from build123d import *

# Parameters (mm, degrees)
SKETCH2_R          = 6.858
EXTRUDE1_DEPTH     = 10.414
EXTRUDE1_DRAFT     = -1.5
CUT_EXTRUDE7_DEPTH = 5.5626


with BuildPart() as part:
    # Sketch2 → Extrude1 (with draft: the straight prism first)
    with BuildSketch(Plane(origin=(-5.207, 0, 0), x_dir=(0, 0, -1), z_dir=(1, 0, 0))):
        Circle(SKETCH2_R)
    extrude(amount=EXTRUDE1_DEPTH)
    # Extrude1: the draft: its side faces are tilted about the plane it starts from
    extrude1_sides = [part.faces().sort_by_distance(p)[0] for p in [
        (0, 0, 6.858),
    ]]
    draft(extrude1_sides, Plane(origin=(-5.207, 0, 0), x_dir=(0, 0, -1), z_dir=(1, 0, 0)), EXTRUDE1_DRAFT)

    # Sketch6 → Cut-Extrude7 (cut)
    with BuildSketch(Plane(origin=(5.207, 0, 0), x_dir=(0, 0, -1), z_dir=(1, 0, 0))):
        Polygon((0, 3.666174209), (-3.175, 1.833087105), (-3.175, -1.833087105), (0, -3.666174209), (3.175, -1.833087105), (3.175, 1.833087105), align=None)
    extrude(amount=-CUT_EXTRUDE7_DEPTH, mode=Mode.SUBTRACT)


solid = part.part
Can you work these out from the model? Positions are in its coordinate system, mm. A direction names the side the tool comes from. Give positions to 0.01 mm unless a question says otherwise; leave off trailing zeros. Order: outer loops, then holes, each group sorted by start corner. A loop starts at its lowest first (then second) coordinate and runs counter-clockwise, first axis right, second up. Notation, with made-up numbers: M 67,65.25 L 86,65.25 A16 ccw 86,92.25 Z; hole C 77.5,-7 d7. An arc over 180 degrees is marked long. Use a Markdown table: item, result. Add a question column.
Item 1: For faces 5 (the flat face through (2, 0, -3.175)), 6 (the flat face through (5.207, -3.1, -1.5)), which set-ups out of +Z, -Z, +X, -X, +Y, -Y let a thin tool reach every point of the face, with its end or its side?
Item 2: Suppose I cut it at D-D (x = -1.5). List the corners of the cut face in (y, z) for me, then the cut area to 3 significant figures.
Item 3: Suppose I cut it at C-C (x = -3). List the corners of the cut face in (y, z) for me.
Item 4: Suppose I cut it at B-B (x = 2). List the corners of the cut face in (y, z) for me (3 decimals).
Item 5: Suppose I cut it at A-A (y = 0). List the corners of the cut face in (x, z) for me (3 decimals), then the cut area to 3 significant figures.
Item 6: We'd pull the mould along Z, two halves only. Please class faces 1 (the flat face through (-5.207, 0, 0)), 2 (the flat face through (2.46, 2.76, 1.57)), 3 (the conical face through (-0.073, -6.826, 1.516)), 4 (the flat face through (2, 0, 3.175)): +Z half, -Z half, draft (parallel to the pull), parting line (faces both ways), or undercut.
Item 7: If I drill on L1, parallel to X at y = 0.5, z = 2.75; L2, parallel to Z at x = 4, y = 1 (3 decimals); L3, parallel to Y at x = 1, z = -2, over which ranges is the centre line in solid material (lowest first)? Write a range as [from, to].
Item 8: Will these pins go through, and if not, where does the flat tip stop? pin 1 (1.5 mm diameter, centred on x = -1, z = 2.5, fed in from -Y); pin 2 (1.5 mm diameter, centred on x = -3, z = 0, fed in from +Y); pin 3 (4 mm diameter, centred on x = 2, z = -2.5, fed in from +Y).
Answer sheet:
| question | item | result |
|---|---|---|
| 1 | face 5 | +X |
| 1 | face 6 | +Z, -Z, +X, +Y, -Y |
| 2 | outline | C 0,0 d13.91 |
| 2 | area | 152 mm² |
| 3 | outline | C 0,0 d13.83 |
| 4 | outline | C 0,0 d14.093; hole M -3.666,0 L -1.833,-3.175 L 1.833,-3.175 L 3.666,0 L 1.833,3.175 L -1.833,3.175 Z |
| 5 | outline | M -5.207,-6.858 L 5.207,-7.131 L 5.207,-3.175 L -0.356,-3.175 L -0.356,3.175 L 5.207,3.175 L 5.207,7.131 L -5.207,6.858 Z |
| 5 | area | 110 mm² |
| 6 | face 1 | draft |
| 6 | face 2 | undercut |
| 6 | face 3 | parting line |
| 6 | face 4 | undercut |
| 7 | L1 | x = [-5.21, -0.36] |
| 7 | L2 | z = [-7.028, -3.175], [3.175, 7.028] |
| 7 | L3 | y = [-6.73, -2.51], [2.51, 6.73] |
| 8 | pin 1 | stops at y = -6.75 |
| 8 | pin 2 | stops at y = 6.94 |
| 8 | pin 3 | stops at y = 7.04 |
